Answer from the drawing. Dimensions are ordinates in mm from the lowest x, y and z of the part. Give positions to 0.01 mm unless a question says otherwise; leave off trailing zeros. Write each loop counter-clockwise with the first axis right and the second up, starting at its lowest first coordinate (ties: lowest second). Pieces come first, ordered by that corner, then holes. Notation, with made-up numbers: (65, 1.25) -> (94, 1.25) arc R11 ccw to (94, 8.25) -> close; hole circle Ø9 at (72.5, 87). An arc over 180 degrees is marked (long way). Put each result on its own line as item: value. Start each with the question number.
1) A cutting plane is placed at D-D (y = 4.5). Write down the section's boundary in (x, z), then the cut area to 3 significant figures.
2) A cutting plane is placed at C-C (z = 1.85). Write down the section's boundary in (x, y).
3) A flat-ended cylindrical pin translates along its axis: pin 1 Ø1.5 at (y, z) = (8, 2) entering from -X. Find the tip coordinate at first contact, or state that the pin passes through.
4) A cutting plane is placed at A-A (x = 5.5). Write down the section's boundary in (y, z), then the cut area to 3 significant figures.
5) A cutting plane is placed at B-B (y = 29.3). Write down the section's boundary in (x, z).
6) Find the intervals of material crossed by line 1 along X through (y, z) = (4.5, 1.25); line 2 along Y through (x, z) = (46.5, 0.85); line 3 along X through (y, z) = (29.3, 1.55), in increasing order. Write a range as from..to.
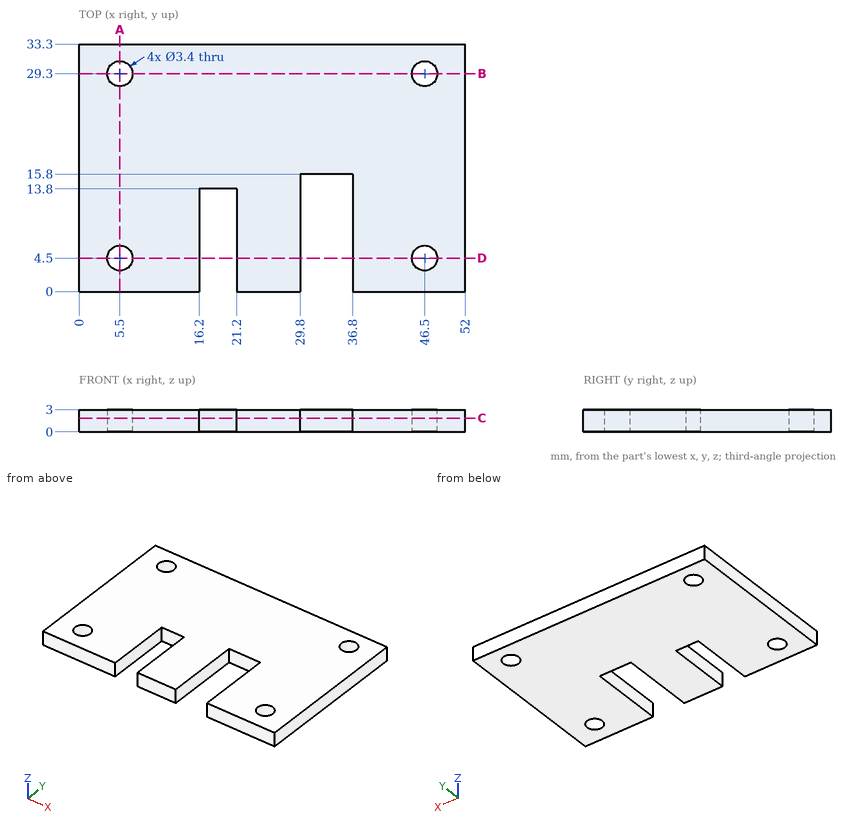
Reply:
1. outline: (0, 0) -> (3.8, 0) -> (3.8, 3) -> (0, 3) -> close; (7.2, 0) -> (16.2, 0) -> (16.2, 3) -> (7.2, 3) -> close; (21.2, 0) -> (29.8, 0) -> (29.8, 3) -> (21.2, 3) -> close; (36.8, 0) -> (44.8, 0) -> (44.8, 3) -> (36.8, 3) -> close; (48.2, 0) -> (52, 0) -> (52, 3) -> (48.2, 3) -> close
1. area: 99.6 mm2
2. outline: (0, 0) -> (16.2, 0) -> (16.2, 13.8) -> (21.2, 13.8) -> (21.2, 0) -> (29.8, 0) -> (29.8, 15.8) -> (36.8, 15.8) -> (36.8, 0) -> (52, 0) -> (52, 33.3) -> (0, 33.3) -> close; hole circle Ø3.4 at (5.5, 4.5); hole circle Ø3.4 at (5.5, 29.3); hole circle Ø3.4 at (46.5, 4.5); hole circle Ø3.4 at (46.5, 29.3)
3. pin 1: stops at x = 0
4. outline: (0, 0) -> (2.8, 0) -> (2.8, 3) -> (0, 3) -> close; (6.2, 0) -> (27.6, 0) -> (27.6, 3) -> (6.2, 3) -> close; (31, 0) -> (33.3, 0) -> (33.3, 3) -> (31, 3) -> close
4. area: 79.5 mm2
5. outline: (0, 0) -> (3.8, 0) -> (3.8, 3) -> (0, 3) -> close; (7.2, 0) -> (44.8, 0) -> (44.8, 3) -> (7.2, 3) -> close; (48.2, 0) -> (52, 0) -> (52, 3) -> (48.2, 3) -> close
6. line 1: x = 0..3.8, 7.2..16.2, 21.2..29.8, 36.8..44.8, 48.2..52
6. line 2: y = 0..2.8, 6.2..27.6, 31..33.3
6. line 3: x = 0..3.8, 7.2..44.8, 48.2..52
